Geometry: final body of the model. Coordinates: model frame, mm. Face numbers are marked on the shaded views. A direction names the side the tool comes from. Round coordinates to 2 decimals unless told otherwise and drop trailing zeros. Loops run counter-clockwise (first coordinate to the right, second up) from the corner with the lowest first, then second, coordinate; pieces in that order, holes last. Notation, with made-up numbers: (-36.5, -20) - (7.5, -20) arc R15 cw to (7.5, -13) - close; hole circle Ø3 at (-13.5, -31.5). An arc over 180 degrees is marked (long way). Answer in a Markdown table with one row per item. Add a question column.
from build123d import *
from OCP.BRepFilletAPI import BRepFilletAPI_MakeChamfer

# Parameters (mm, degrees)
SKETCH1_W           = 18
SKETCH1_H           = 18
BOSS_EXTRUDE1_DEPTH = 25
CIRPATTERN1_COUNT   = 5
CIRPATTERN1_ANGLE   = 160
CHAMFER1_SIZE       = 15
CHAMFER1_SIZE2      = 8.660254038
CHAMFER2_SIZE       = 10
CHAMFER2_SIZE2      = 5.773502692
CHAMFER3_SIZE       = 4
CHAMFER3_SIZE2      = 6.92820323


with BuildPart() as part:
    # Sketch1 → Boss-Extrude1 (new body)
    with BuildSketch(Plane.XY):
        with BuildLine():
            Line((-119, 0), (0, 0))
            ThreePointArc((0, 0), (-59.5, -59.5), (-119, 0))
        make_face()
        with Locations((-40, -24)):
            Rectangle(SKETCH1_W, SKETCH1_H, mode=Mode.SUBTRACT)
        with Locations((-79, -24)):
            Rectangle(SKETCH1_W, SKETCH1_H, mode=Mode.SUBTRACT)
    extrude(amount=BOSS_EXTRUDE1_DEPTH)

    # Sketch4 → Ø4.0mm Dowel Hole2 (revolve, cut)
    with BuildSketch(Plane(origin=(-0.903938696, -10.332066571, 12.5), x_dir=(0.1736481776669305, 0.9848077530122081, 0), z_dir=(0, 0, 1))):
        Polygon((0, 0), (0, 11.201721238), (2, 10), (2, 0.025), (2.025, 0), align=None)
    f_4_0mm_dowel_hole2 = revolve(axis=Axis((5.349590536, -11.434732499, 12.5), (-0.9848077530122081, 0.1736481776669305, 0)), mode=Mode.SUBTRACT)

    # CirPattern1: Ø4.0mm Dowel Hole2 ×5 about axis
    cirpattern1_axis = Axis((-59.5, 0, 0), (0, 0, -1))
    for i in range(1, CIRPATTERN1_COUNT):
        add(f_4_0mm_dowel_hole2.rotate(cirpattern1_axis, i * CIRPATTERN1_ANGLE / (CIRPATTERN1_COUNT - 1)), mode=Mode.SUBTRACT)

    # Chamfer1: one chamfer whose edges measure the first distance from different faces: ONE call of the kernel's chamfer builder (chamfer() names one face for all edges)
    chamfer1_edges_1 = [part.edges().sort_by_distance(p)[0] for p in [
        (-40, -15, 25),
    ]]
    chamfer1_side_1 = [part.faces().sort_by_distance(p)[0] for p in [
        (-40, -15, 12.5),
    ]]
    chamfer1_edges_2 = [part.edges().sort_by_distance(p)[0] for p in [
        (-79, -15, 25),
    ]]
    chamfer1_side_2 = [part.faces().sort_by_distance(p)[0] for p in [
        (-79, -15, 12.5),
    ]]
    chamfer1 = BRepFilletAPI_MakeChamfer(part.part.solid().wrapped)
    for e in chamfer1_edges_1:
        chamfer1.Add(CHAMFER1_SIZE, CHAMFER1_SIZE2, e.wrapped, chamfer1_side_1[0].wrapped)  # the first distance lies on this face
    for e in chamfer1_edges_2:
        chamfer1.Add(CHAMFER1_SIZE, CHAMFER1_SIZE2, e.wrapped, chamfer1_side_2[0].wrapped)  # the first distance lies on this face
    add(Compound.cast(chamfer1.Shape()), mode=Mode.REPLACE)

    # Chamfer2: one chamfer whose edges measure the first distance from different faces: ONE call of the kernel's chamfer builder (chamfer() names one face for all edges)
    chamfer2_edges_1 = [part.edges().sort_by_distance(p)[0] for p in [
        (-49, -24, 0),
    ]]
    chamfer2_side_1 = [part.faces().sort_by_distance(p)[0] for p in [
        (-49, -22.500700474, 13.445989877),
    ]]
    chamfer2_edges_2 = [part.edges().sort_by_distance(p)[0] for p in [
        (-31, -24, 0),
    ]]
    chamfer2_side_2 = [part.faces().sort_by_distance(p)[0] for p in [
        (-31, -22.500700474, 13.445989877),
    ]]
    chamfer2_edges_3 = [part.edges().sort_by_distance(p)[0] for p in [
        (-88, -24, 0),
    ]]
    chamfer2_side_3 = [part.faces().sort_by_distance(p)[0] for p in [
        (-88, -22.500700474, 13.445989877),
    ]]
    chamfer2_edges_4 = [part.edges().sort_by_distance(p)[0] for p in [
        (-70, -24, 0),
    ]]
    chamfer2_side_4 = [part.faces().sort_by_distance(p)[0] for p in [
        (-70, -22.500700474, 13.445989877),
    ]]
    chamfer2 = BRepFilletAPI_MakeChamfer(part.part.solid().wrapped)
    for e in chamfer2_edges_1:
        chamfer2.Add(CHAMFER2_SIZE, CHAMFER2_SIZE2, e.wrapped, chamfer2_side_1[0].wrapped)  # the first distance lies on this face
    for e in chamfer2_edges_2:
        chamfer2.Add(CHAMFER2_SIZE, CHAMFER2_SIZE2, e.wrapped, chamfer2_side_2[0].wrapped)  # the first distance lies on this face
    for e in chamfer2_edges_3:
        chamfer2.Add(CHAMFER2_SIZE, CHAMFER2_SIZE2, e.wrapped, chamfer2_side_3[0].wrapped)  # the first distance lies on this face
    for e in chamfer2_edges_4:
        chamfer2.Add(CHAMFER2_SIZE, CHAMFER2_SIZE2, e.wrapped, chamfer2_side_4[0].wrapped)  # the first distance lies on this face
    add(Compound.cast(chamfer2.Shape()), mode=Mode.REPLACE)

    # Chamfer3
    chamfer3_edges = [part.edges().sort_by_distance(p)[0] for p in [
        (-40, -15, 0),
        (-79, -15, 0),
    ]]
    chamfer3_side = [part.faces().sort_by_distance(p)[0] for p in [
        (-59.5, -25.548841696, 0),
    ]]
    chamfer(chamfer3_edges, length=CHAMFER3_SIZE, length2=CHAMFER3_SIZE2, reference=chamfer3_side[0])


solid = part.part
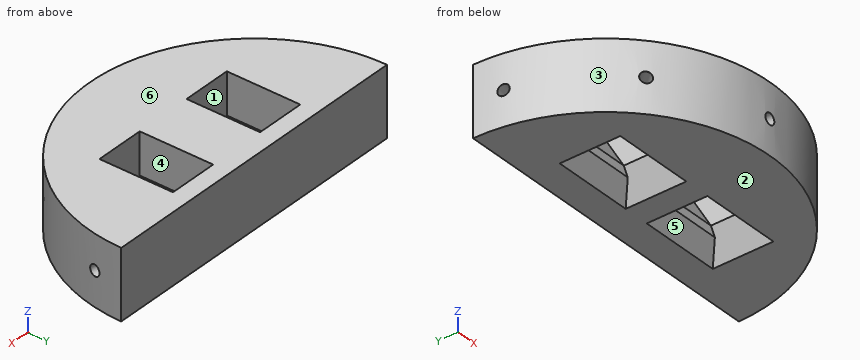
1) Section B-B, the plane x = -84.5. Return the cut outline in (y, z).
2) Section A-A, the plane y = -23. Return the cut outline in (x, z), and give its area (3 significant figures).
3) Contact query for flat-ended pins moving along their axis: pin 1 Ø7.5 at (y, z) = (-26, 14) entering from -X; pin 2 Ø7.5 at (y, z) = (-25, 15) entering from +X; pin 3 Ø5 at (y, z) = (-31, 3) entering from +X; pin 4 Ø4 at (x, y) = (-105.5, -23.5) entering from -Z. Output: stop coordinate, or through.
4) Pull-direction query (Y, two-part tool) for the marked faces 1, 2 and 3; classes: pulls with the +Y half, pulls with the -Y half, needs draft (parallel to the pull), parting line crosses it, or undercut.
5) Section D-D, the plane x = -33. Return the cut outline in (y, z), and give its area (3 significant figures).
6) Reachability of the marked faces 4, 5 and 6 from +Z, -Z, +X, -X, +Y, -Y: full face, straight path, thin tool, end or side. Return the list, or none.
7) Material intervals for line 1 along Z through (x, y) = (-59.5, -52.75); line 2 along X through (y, z) = (-19, 12.25); line 3 along Y through (x, z) = (-74, 2.5), sorted ascending. Write a range as from..to.
8) Section C-C, the plane y = -53. Return the cut outline in (x, z), and give its area (3 significant figures).
Evaluation:
| question | item | result |
|---|---|---|
| 1 | outline | (-53.99, 0) - (-33, 0) - (-33, 25) - (-53.99, 25) - close; (-15, 6.93) - (-11, 0) - (0, 0) - (0, 25) - (-6.34, 25) - (-15, 10) - close |
| 2 | outline | (-114.37, 0) - (-93.77, 0) - (-88, 10) - (-88, 25) - (-114.37, 25) - close; (-70, 10) - (-64.23, 0) - (-54.77, 0) - (-49, 10) - (-49, 25) - (-70, 25) - close; (-31, 10) - (-25.23, 0) - (-4.63, 0) - (-4.63, 25) - (-31, 25) - close |
| 2 | area | 1,730 mm² |
| 3 | pin 1 | stops at x = -114.68 |
| 3 | pin 2 | stops at x = -3.92 |
| 3 | pin 3 | stops at x = -7.27 |
| 3 | pin 4 | stops at z = 0 |
| 4 | face 1 | undercut |
| 4 | face 2 | needs draft |
| 4 | face 3 | pulls with the -Y half |
| 5 | outline | (-53.27, 0) - (-33, 0) - (-33, 25) - (-53.27, 25) - close; (-15, 6.93) - (-11, 0) - (0, 0) - (0, 25) - (-6.34, 25) - (-15, 10) - close |
| 5 | area | 803 mm² |
| 6 | face 4 | +Z |
| 6 | face 5 | -Z |
| 6 | face 6 | +Z, +X, -X, +Y, -Y |
| 7 | line 1 | z = 0..10.5, 14.5..25 |
| 7 | line 2 | x = -115.88..-88, -70..-49, -31..-3.12 |
| 7 | line 3 | y = -57.71..-33, -12.44..0 |
| 8 | outline | (-86.54, 0) - (-32.46, 0) - (-32.46, 25) - (-86.54, 25) - close; hole circle Ø4 at (-59.5, 12.5) |
| 8 | area | 1,340 mm² |
